Read the model definition and answer for the solid it produces. Units are mm, in the model's axes. Coordinates: 2 decimals unless noted, no trailing zeros. Write each loop counter-clockwise with the first axis right and the second up, starting at its lowest first coordinate (ties: lowest second). Pieces come first, ordered by that corner, then holes. Notation, with made-up numbers: (21.25, 1.25) - (73.25, 1.25) arc R12 ccw to (73.25, 22.25) - close; hole circle Ø8 at (49.5, 48.25). An arc over 180 degrees is marked (long way). Return JSON: item names as keys, results as strings.
```python
from build123d import *

# Parameters (mm, degrees)
SKETCH_R           = 50
SKETCH_R_2         = 16
PAD_DEPTH          = 2
SKETCH001_R        = 1.25
POCKET_DEPTH       = 282.871995
POCKET_DEPTH_BACK  = 284.871995
POLARPATTERN_COUNT = 8


with BuildPart() as part:
    # Sketch → Pad (new body)
    with BuildSketch(Plane.XY):
        Circle(SKETCH_R)
        Circle(SKETCH_R_2, mode=Mode.SUBTRACT)
    extrude(amount=PAD_DEPTH)

    # Sketch001 → Pocket (cut, two sides)
    with BuildSketch(Plane.XY) as pocket_sk:
        with Locations((24, 0)):
            Circle(SKETCH001_R)
        with Locations((42, 0)):
            Circle(SKETCH001_R)
    pocket = extrude(amount=-POCKET_DEPTH, mode=Mode.SUBTRACT) + extrude(pocket_sk.sketch, amount=POCKET_DEPTH_BACK, mode=Mode.SUBTRACT)

    # PolarPattern: Pocket ×8 about axis
    polarpattern_axis = Axis((0, 0, 0), (0, 0, 1))
    for i in range(1, POLARPATTERN_COUNT):
        add(pocket.rotate(polarpattern_axis, i * 360 / POLARPATTERN_COUNT), mode=Mode.SUBTRACT)


solid = part.part
```
(1) Determine the mould class of faces 1 (the face through (-0.05, 40.75, 1.01)), 2 (the face through (-12, 12, 2)), 3 (the face through (47.69, 15.02, 0.99)) for opening direction Y: +Y half, -Y half, draft (parallel to the pull), parting line (faces both ways), or undercut.
Answer:
{"face 1": "undercut", "face 2": "draft", "face 3": "parting line"}
(2) A cutting plane is placed at C-C (y = -42). Determine the outline of the cut face in (x, z), and give its area (3 significant figures).
Answer:
{"outline": "(-27.13, 0) - (-1.25, 0) - (-1.25, 2) - (-27.13, 2) - close; (1.25, 0) - (27.13, 0) - (27.13, 2) - (1.25, 2) - close", "area": "104 mm²"}
(3) A cutting plane is placed at A-A (y = 0). Determine the outline of the cut face in (x, z).
Answer:
{"outline": "(-50, 0) - (-43.25, 0) - (-43.25, 2) - (-50, 2) - close; (-40.75, 0) - (-25.25, 0) - (-25.25, 2) - (-40.75, 2) - close; (-22.75, 0) - (-16, 0) - (-16, 2) - (-22.75, 2) - close; (16, 0) - (22.75, 0) - (22.75, 2) - (16, 2) - close; (25.25, 0) - (40.75, 0) - (40.75, 2) - (25.25, 2) - close; (43.25, 0) - (50, 0) - (50, 2) - (43.25, 2) - close"}
(4) A cutting plane is placed at D-D (x = -24). Determine the outline of the cut face in (y, z).
Answer:
{"outline": "(-43.86, 0) - (-1.25, 0) - (-1.25, 2) - (-43.86, 2) - close; (1.25, 0) - (43.86, 0) - (43.86, 2) - (1.25, 2) - close"}
(5) Straight lines are drawn through the part: line 1 (Y direction, x = 16.5, z = 0.55); line 2 (Y direction, x = 1, z = 1.05); line 3 (X direction, y = -24, z = 0.3). For each, find the intervals that lie inside material, in ascending order. Write a range as from..to.
Answer:
{"line 1": "-47.2..-18.13, -15.81..15.81, 18.13..47.2", "line 2": "-49.99..-42.75, -41.25..-24.75, -23.25..-15.97, 15.97..23.25, 24.75..41.25, 42.75..49.99", "line 3": "-43.86..-1.25, 1.25..43.86"}
(6) Flat-ended cylindrical pins translate along their axes: P1, Ø2, axis at x = -29.7, y = -29.7, coming from the +Z side (3 decimals); P2, Ø1, axis at y = -34.5, z = 2, coming from the +X side. Find the tip coordinate at first contact, or state that the pin passes through.
Answer:
{"P1": "through", "P2": "x = 36.66"}
